from build123d import *

# Parameters (mm, degrees)
SKETCH1_R           = 11.938
SKETCH1_R_2         = 8.763
BOSS_EXTRUDE1_DEPTH = 5.08
SKETCH2_R           = 11.938
BOSS_EXTRUDE2_DEPTH = 2.54
BOSS_EXTRUDE6_DEPTH = 2.54


with BuildPart() as part:
    # Sketch1 → Boss-Extrude1 (new body)
    with BuildSketch(Plane.XY):
        Circle(SKETCH1_R)
        Circle(SKETCH1_R_2, mode=Mode.SUBTRACT)
    extrude(amount=BOSS_EXTRUDE1_DEPTH)

    # Sketch2 → Boss-Extrude2 (add)
    with BuildSketch(Plane.XY.offset(5.08)):
        Circle(SKETCH2_R)
    extrude(amount=BOSS_EXTRUDE2_DEPTH)

    # Sketch3 → Boss-Extrude6 (add)
    with BuildSketch(Plane.XY.offset(7.62)):
        with BuildLine():
            Line((-3.678678712, -5.714068812), (-3.678678712, -4.50574791))
            ThreePointArc((-3.678678712, -4.50574791), (-2.295527202, -1.765380595), (-1.819182511, 1.267079934))
            Line((-1.819182511, 1.267079934), (-1.819182511, 2.8590046))
            Line((-1.819182511, 2.8590046), (-3.070257362, 2.8590046))
            Line((-3.070257362, 2.8590046), (-3.070257362, 4.076695904))
            Line((-3.070257362, 4.076695904), (-2.383695529, 4.076695904))
            ThreePointArc((-2.383695529, 4.076695904), (-2.843426725, 4.797347732), (-3.070257362, 5.621507725))
            Line((-3.070257362, 5.621507725), (-3.070257362, 6.406088041))
            ThreePointArc((-3.070257362, 6.406088041), (-2.815803075, 6.808897948), (-2.383695529, 7.00961136))
            Line((-2.383695529, 7.00961136), (-0.612171184, 7.15577449))
            Line((-0.612171184, 7.15577449), (-0.612171184, 7.768514842))
            Line((-0.612171184, 7.768514842), (-1.220124502, 7.768514842))
            Line((-1.220124502, 7.768514842), (-1.220124502, 8.998782581))
            Line((-1.220124502, 8.998782581), (-0.612171184, 8.998782581))
            Line((-0.612171184, 8.998782581), (-0.612171184, 9.616309967))
            Line((-0.612171184, 9.616309967), (0.612171184, 9.616309967))
            Line((0.612171184, 9.616309967), (0.612171184, 8.998782581))
            Line((0.612171184, 8.998782581), (1.220124502, 8.998782581))
            Line((1.220124502, 8.998782581), (1.220124502, 7.768514842))
            Line((1.220124502, 7.768514842), (0.612171184, 7.768514842))
            Line((0.612171184, 7.768514842), (0.612171184, 7.15577449))
            Line((0.612171184, 7.15577449), (2.383695529, 7.00961136))
            ThreePointArc((2.383695529, 7.00961136), (2.815803075, 6.808897948), (3.070257362, 6.406088041))
            Line((3.070257362, 6.406088041), (3.070257362, 5.621507725))
            ThreePointArc((3.070257362, 5.621507725), (2.843426725, 4.797347732), (2.383695529, 4.076695904))
            Line((2.383695529, 4.076695904), (3.070257362, 4.076695904))
            Line((3.070257362, 4.076695904), (3.070257362, 2.8590046))
            Line((3.070257362, 2.8590046), (1.819182511, 2.8590046))
            Line((1.819182511, 2.8590046), (1.819182511, 1.267079934))
            ThreePointArc((1.819182511, 1.267079934), (2.295527202, -1.765380595), (3.678678712, -4.50574791))
            Line((3.678678712, -4.50574791), (3.678678712, -5.714068812))
            Line((3.678678712, -5.714068812), (4.863085817, -5.714068812))
            Line((4.863085817, -5.714068812), (4.863085817, -8.173503524))
            Line((4.863085817, -8.173503524), (-4.920042397, -8.173503524))
            Line((-4.920042397, -8.173503524), (-4.920042397, -5.714068812))
            Line((-4.920042397, -5.714068812), (-3.678678712, -5.714068812))
        make_face()
    extrude(amount=BOSS_EXTRUDE6_DEPTH)


solid = part.part
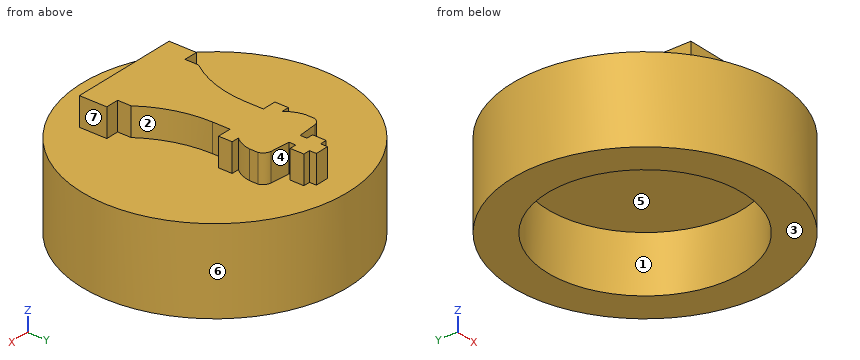
Geometry check sheet. Reference: the model listing, model coordinates, mm. Face numbers are marked on the shaded views. A direction names the side the tool comes from. Round coordinates to 2 decimals unless told otherwise and drop trailing zeros. Loops run counter-clockwise (first coordinate to the right, second up) from the corner with the lowest first, then second, coordinate; pieces in that order, holes last. Notation, with made-up numbers: (-38.5, 37) -> (18.5, 37) arc R16 cw to (18.5, 46) -> close; hole circle Ø9 at (42.25, 66.25). An arc over 180 degrees is marked (long way). Answer as a JSON object with one key per item and string values. Group by question number.
Item 1: Cross-section at D-D, the plane z = 6.5. Record the cut outline in (x, y), plus the area to 3 significant figures.
Item 2: Release check for a two-part mould opening along Y. For the marked faces 4, 5, 6 and 7 record: pulls with the +Y half, pulls with the -Y half, needs draft (parallel to the pull), parting line crosses it, or undercut.
Item 3: Cross-section at B-B, the plane z = 4.5. Record the cut outline in (x, y).
Item 4: Depth check by flat-ended pin: pin 1 Ø1.5 at (x, z) = (-8.5, 2.5) entering from -Y; pin 2 Ø2 at (x, z) = (1.5, 5.5) entering from -Y; pin 3 Ø2 at (x, z) = (2.5, 6) entering from -Y. Enter the tip coordinate at first touch or a pass-through.
Item 5: Cross-section at C-C, the plane y = 0. Record the cut outline in (x, z).
Item 6: Set-up check for the marked faces 1, 2 and 3: record each of +Z, -Z, +X, -X, +Y, -Y from which the full face is reachable in a straight line by a thin tool's end or side.
Item 7: Cross-section at A-A, the plane x = 0. Record the cut outline in (y, z), plus the area to 3 significant figures.
Item 8: Thickness scan on line 1 along Y through (x, z) = (0, 1.6); line 2 along Z through (x, y) = (-3.5, -5); line 3 along Z through (x, y) = (-3, -1.75). Record the ranges inside material, lowest first.
Determined:
{
 "1": {"outline": "circle Ø23.88 at (0, 0)", "area": "448 mm²"},
 "2": {"face 4": "undercut", "face 5": "undercut", "face 6": "parting line crosses it", "face 7": "needs draft"},
 "3": {"outline": "circle Ø23.88 at (0, 0); hole circle Ø17.53 at (0, 0)"},
 "4": {"pin 1": "stops at y = -9.08", "pin 2": "stops at y = -11.93", "pin 3": "stops at y = -11.84"},
 "5": {"outline": "(-11.94, 0) -> (-8.76, 0) -> (-8.76, 5.08) -> (8.76, 5.08) -> (8.76, 0) -> (11.94, 0) -> (11.94, 7.62) -> (1.9, 7.62) -> (1.9, 10.16) -> (-1.9, 10.16) -> (-1.9, 7.62) -> (-11.94, 7.62) -> close"},
 "6": {"face 1": "-Z", "face 2": "+Z, +X", "face 3": "-Z, +X, -X, +Y, -Y"},
 "7": {"outline": "(-11.94, 0) -> (-8.76, 0) -> (-8.76, 5.08) -> (8.76, 5.08) -> (8.76, 0) -> (11.94, 0) -> (11.94, 7.62) -> (9.62, 7.62) -> (9.62, 10.16) -> (-8.17, 10.16) -> (-8.17, 7.62) -> (-11.94, 7.62) -> close", "area": "138 mm²"},
 "8": {"line 1": "y = -11.94 to -8.76, 8.76 to 11.94", "line 2": "z = 5.08 to 10.16", "line 3": "z = 5.08 to 7.62"}
}
